Source: CAD feature listing. Evaluate the final solid. Frame: model axes, mm. Give positions to 0.01 mm unless a question says otherwise; leave off trailing zeros. Loops run counter-clockwise (first coordinate to the right, second up) from the corner with the lowest first, then second, coordinate; pieces in that order, holes last. Notation, with made-up numbers: (43, 28.5) - (61, 28.5) arc R36 cw to (61, 66.5) - close; hole circle Ø8 at (21.5, 8.5). An arc over 180 degrees is marked (long way). Write each question's results on one line, items separated by ' | '. Start each with the question number.
(1) Cut plane C-C on y = 62. Return the cut outline in (x, z) (3 decimals), then the cut area to 3 significant figures.
(2) Cut plane B-B on x = -1.15. Return the cut outline in (y, z).
(3) Material intervals for line 1 along X through (y, z) = (29, -0.15); line 2 along X through (y, z) = (47, -0.9); line 3 along Z through (x, y) = (-0.5, 31.5), sorted ascending. Write a range as [from, to].
(4) Cut plane A-A on z = 1.25. Return the cut outline in (x, y), then the cut area to 3 significant figures.
(5) Contact query for flat-ended pins moving along their axis: pin 1 (1 mm diameter, centred on y = 10, z = 0.5, fed in from +X); pin 2 (0.5 mm diameter, centred on x = 2, y = 62.5, fed in from +Z); pin 3 (1 mm diameter, centred on y = 61.5, z = 0, fed in from +X). Output: stop coordinate, or through.
from build123d import *

# Parameters (mm, degrees)
SKETCH1_R           = 2.5
BOSS_EXTRUDE1_DEPTH = 70
SKETCH2_W           = 8.002740347
SKETCH2_H           = 0.39
SKETCH3_W           = 11.814730857
SKETCH3_H           = 0.39
SKETCH4_W           = 12.637510598
SKETCH4_H           = 0.39
CUT_EXTRUDE1_DEPTH  = 0.7
SKETCH6_W           = 1.25
SKETCH6_H           = 31.626867322
CUT_EXTRUDE2_DEPTH  = 0.7


with BuildPart() as part:
    # Sketch1 → Boss-Extrude1 (new body)
    with BuildSketch(Plane(origin=(0, 0, 0), x_dir=(1, 0, 0), z_dir=(0, 1, 0))):
        with Locations(Location((0, 0, 0), (0, 0, 270))):
            Circle(SKETCH1_R)
    extrude(amount=BOSS_EXTRUDE1_DEPTH)

    # Sketch2 → Cut-Revolve1 (revolve, cut)
    with BuildSketch(Plane(origin=(0, 0, 0), x_dir=(0, 0, -1), z_dir=(1, 0, 0))):
        with Locations((-6.341370174, 65.195)):
            Rectangle(SKETCH2_W, SKETCH2_H)
    revolve(axis=Axis((0, 67.145702963, 0), (0, -1, 0)), mode=Mode.SUBTRACT)

    # Sketch3 → Cut-Revolve2 (revolve, cut)
    with BuildSketch(Plane(origin=(0, 0, 0), x_dir=(0, 0, -1), z_dir=(1, 0, 0)), mode=Mode.PRIVATE) as cut_revolve2_sk:
        with Locations((-8.247365429, 59.805)):
            Rectangle(SKETCH3_W, SKETCH3_H)
    revolve(cut_revolve2_sk.sketch.rotate(Axis((0, 61.014608436, 0), (0, -1, 0)), 180), axis=Axis((0, 61.014608436, 0), (0, -1, 0)), mode=Mode.SUBTRACT)

    # Sketch4 → Cut-Revolve3 (revolve, cut)
    with BuildSketch(Plane(origin=(0, 0, 0), x_dir=(0, 0, -1), z_dir=(1, 0, 0)), mode=Mode.PRIVATE) as cut_revolve3_sk:
        with Locations((-8.658755299, 26.915)):
            Rectangle(SKETCH4_W, SKETCH4_H)
    revolve(cut_revolve3_sk.sketch.rotate(Axis((0, 27.341534507, 0), (0, -1, 0)), 180), axis=Axis((0, 27.341534507, 0), (0, -1, 0)), mode=Mode.SUBTRACT)

    # Sketch5 → Cut-Extrude1 (cut)
    with BuildSketch(Plane(origin=(2.5, 0, 0), x_dir=(0, 0, -1), z_dir=(1, 0, 0))):
        with BuildLine():
            Line((0.625, 65), (0.625, 60))
            ThreePointArc((0.625, 60), (0, 59.375), (-0.625, 60))
            Line((-0.625, 60), (-0.625, 65))
            ThreePointArc((-0.625, 65), (0, 65.625), (0.625, 65))
        make_face()
    extrude(amount=-CUT_EXTRUDE1_DEPTH, mode=Mode.SUBTRACT)

    # Sketch6 → Cut-Extrude2 (cut)
    with BuildSketch(Plane(origin=(2.5, 0, 0), x_dir=(0, 0, -1), z_dir=(1, 0, 0))):
        with Locations((0, 10.046566339)):
            Rectangle(SKETCH6_W, SKETCH6_H)
    extrude(amount=-CUT_EXTRUDE2_DEPTH, mode=Mode.SUBTRACT)


solid = part.part
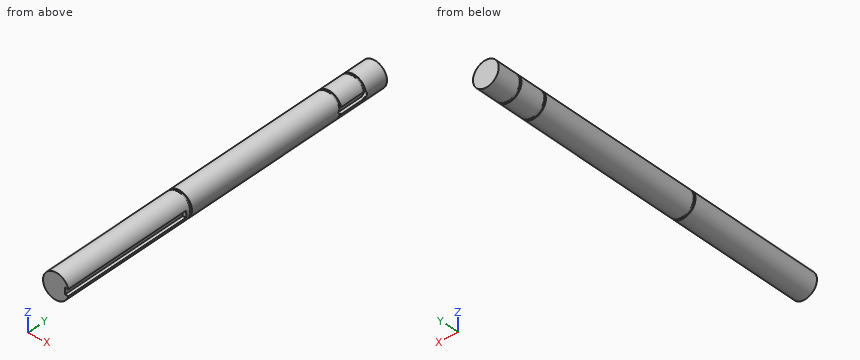
Ans:
1) outline: (1.8, -0.625) - (1.8, 0.625) - (2.421, 0.625) arc R2.5 ccw (long way) to (2.421, -0.625) - close | area: 18.8 mm^2
2) outline: (0, -2.22) - (26.72, -2.22) - (26.72, -2.04) - (27.11, -2.04) - (27.11, -2.22) - (59.61, -2.22) - (59.61, -2.04) - (60, -2.04) - (60, -2.22) - (65, -2.22) - (65, -2.04) - (65.39, -2.04) - (65.39, -2.22) - (70, -2.22) - (70, 2.22) - (65.39, 2.22) - (65.39, 2.04) - (65, 2.04) - (65, 2.22) - (60, 2.22) - (60, 2.04) - (59.61, 2.04) - (59.61, 2.22) - (27.11, 2.22) - (27.11, 2.04) - (26.72, 2.04) - (26.72, 2.22) - (0, 2.22) - close
3) line 1: [-2.5, 2.5] | line 2: [-2.33, 2.33] | line 3: [-2.45, 2.45]
4) outline: (-2.17, 0) - (2.17, 0) - (2.17, 26.72) - (1.98, 26.72) - (1.98, 27.11) - (2.17, 27.11) - (2.17, 59.61) - (1.98, 59.61) - (1.98, 60) - (2.17, 60) - (2.17, 65) - (1.98, 65) - (1.98, 65.39) - (2.17, 65.39) - (2.17, 70) - (-2.17, 70) - (-2.17, 65.39) - (-1.98, 65.39) - (-1.98, 65) - (-2.17, 65) - (-2.17, 60) - (-1.98, 60) - (-1.98, 59.61) - (-2.17, 59.61) - (-2.17, 27.11) - (-1.98, 27.11) - (-1.98, 26.72) - (-2.17, 26.72) - close | area: 303 mm^2
5) pin 1: x = 2.42 | pin 2: z = 1.79 | pin 3: x = 1.8
